CAD build for the part. Positions are in the model's coordinates, mm. A direction names the side the tool comes from. Give positions to 0.01 mm unless a question says otherwise; leave off trailing zeros. Order: outer loops, then holes, each group sorted by start corner. A loop starts at its lowest first (then second) coordinate and runs counter-clockwise, first axis right, second up. Notation, with made-up numbers: M 26.25,65 L 61.25,65 A22 cw 61.25,74 Z; hole C 83.5,26.25 d4. An arc over 180 degrees is marked long. Put each result on its own line as item: value. Start each with the question number.
1) Cut at C-C (y = 2.5). Write the cut outline in (x, z), and give its area (3 significant figures).
2) Pin check, flat tips, straight feed: pin 1 (1.7 mm diameter, centred on y = -34.5, z = 2.5, fed in from -X); pin 2 (2 mm diameter, centred on x = 2.5, y = 40, fed in from -Z); pin 3 (0.8 mm diameter, centred on y = 71.5, z = 3.5, fed in from -X). Stop position of each tip, or through.
3) Cut at D-D (y = 58.5). Write the cut outline in (x, z), and give its area (3 significant figures).
4) Two-plate mould, pull along X, no slides. Class faces 5 (the face through (0, -44.6, 0)), 6 (the face through (0, 71, 2.2)), 7 (the face through (1.08, 8.78, 4.88)): released by +X, released by -X, zero draft, split by the parting line, or undercut.
5) Cut at A-A (z = 0). Write the cut outline in (x, y), and give its area (3 significant figures).
6) Cut at B-B (x = 0). Write the cut outline in (y, z).
7) Tool access for faces 1 (the face through (-0.867, 50.387, -3.905)), 2 (the face through (0, 83.9, 0)), 3 (the face through (2.15, -21.988, -3.373)), 4 (the face through (0, -31, 2.2)): list every direction of +Z, -Z, +X, -X, +Y, -Y with a clear straight run to the whole face (end or side of a thin tool).
8) Drill centre lines: line 1 (Y direction, x = 0.25, z = 2.5); line 2 (Y direction, x = 3, z = 3.25); line 3 (X direction, y = -39, z = 3). Where is each one in solid material? Low to high. Write a range as [from, to].
Autodesk Inventor part; units mm, degrees
ref_plane "作業平面1" through (0, -44.6, 4) normal (0, 0, 1) x (1, 0, 0)
ref_plane "YZ Plane" through (0, 0, 0) normal (1, 0, 0) x (0, 1, 0)
ref_plane "XZ Plane" through (0, 0, 0) normal (0, 1, 0) x (-1, 0, 0)
sketch "スケッチ1" plane through (0, 0, 0) normal (0, 1, 0) x (-1, 0, 0)
  circle A0 centre (0, 0) radius 5
  dimension "d0" = 10
extrude "押し出し1" add sketch "スケッチ1" along normal blind 17.8
sketch "スケッチ2" plane through (0, 17.8, 0) normal (0, 1, 0) x (1, 0, 0)
  circle A0 centre (0, 0) radius 4
  dimension "d3" = 8
extrude "押し出し2" add sketch "スケッチ2" along normal blind 66.1
sketch "スケッチ3" plane through (0, 0, 0) normal (0, -1, 0) x (1, 0, 0)
  circle A0 centre (0, 0) radius 4
  dimension "d6" = 8
extrude "押し出し3" add sketch "スケッチ3" along normal blind 44.6
sketch "スケッチ4" plane through (0, -44.6, 0) normal (0, -1, 0) x (1, 0, 0)
  circle A0 centre (0, 0) radius 4
  point P0 (0, 4)
ref_plane "作業平面1" through (0, -44.6, 4) normal (0, 0, 1) x (1, 0, 0)
sketch "スケッチ7" plane through (0, -44.6, 4) normal (0, 0, 1) x (1, 0, 0)
  line L0 (-1.5, 5) -> (1.5, 5)
  line L1 (1.5, 5) -> (1.5, 21)
  line L2 (1.5, 21) -> (-1.5, 21)
  line L3 (-1.5, 21) -> (-1.5, 5)
  line L4 (-1.5, 5) -> (1.5, 21) construction
  line L5 (1.5, 5) -> (-1.5, 21) construction
  line L6 (-4, 0) -> (4, 0)
  line L7 (-1.5, 107.5) -> (1.5, 107.5)
  line L8 (1.5, 107.5) -> (1.5, 123.5)
  line L9 (1.5, 123.5) -> (-1.5, 123.5)
  line L10 (-1.5, 123.5) -> (-1.5, 107.5)
  line L11 (-1.5, 107.5) -> (1.5, 123.5) construction
  line L12 (1.5, 107.5) -> (-1.5, 123.5) construction
  line L13 (4, 128.5) -> (-4, 128.5)
  point P0 (0, 44.6)
  point P1 (0, 13)
  point P2 (0, 115.5)
  dimension "d17" = 3
  dimension "d18" = 16
  dimension "d19" = 5
  dimension "d20" = 3
  dimension "d21" = 16
  dimension "d22" = 5
extrude "押し出し5" cut sketch "スケッチ7" against normal blind 1.8
properties part number "shoulder2_shaft2" material "鋼、炭素鋼"
Solution:
1. outline: C 0,0 d10
1. area: 78.5 mm²
2. pin 1: x = -3.64
2. pin 2: z = -3.71
2. pin 3: x = -2.53
3. outline: C 0,0 d8
3. area: 50.3 mm²
4. face 5: zero draft
4. face 6: undercut
4. face 7: split by the parting line
5. outline: M -5,0 L -4,0 L -4,-44.6 L 4,-44.6 L 4,0 L 5,0 L 5,17.8 L 4,17.8 L 4,83.9 L -4,83.9 L -4,17.8 L -5,17.8 Z
5. area: 1,060 mm²
6. outline: M -44.6,-4 L 0,-4 L 0,-5 L 17.8,-5 L 17.8,-4 L 83.9,-4 L 83.9,4 L 78.9,4 L 78.9,2.2 L 62.9,2.2 L 62.9,4 L 17.8,4 L 17.8,5 L 0,5 L 0,4 L -23.6,4 L -23.6,2.2 L -39.6,2.2 L -39.6,4 L -44.6,4 Z
7. face 1: +Y
7. face 2: +Z, -Z, +X, -X, +Y
7. face 3: -Y
7. face 4: +Z
8. line 1: [-44.6, -39.6], [-23.6, 62.9], [78.9, 83.9]
8. line 2: [0, 17.8]
8. line 3: [-2.65, -1.5], [1.5, 2.65]
